```python
from build123d import *

# Parameters (mm, degrees)
F0_R     = 11
F1_DEPTH = 3.5
F2_R     = 5
F3_DEPTH = 1.5
F4_R     = 5
F5_DEPTH = 10
F6_R     = 4
F7_DEPTH = 25.4
F8_R     = 1.75
F9_DEPTH = 25.4
F10_SIZE = 0.381
F11_SIZE = 0.381


with BuildPart() as f1:
    # F0 (on Front) → F1 (new body)
    with BuildSketch(Plane.XZ):
        Circle(F0_R)
    extrude(amount=F1_DEPTH)

    # F2 (on face) → F3 (join)
    with BuildSketch(Plane.XZ.offset(3.5)):
        Circle(F2_R)
    extrude(amount=F3_DEPTH)

    # F4 (on face) → F5 (join)
    with BuildSketch(Plane(origin=(0, 0, 0), x_dir=(-1, 0, 0), z_dir=(0, 1, 0))):
        Circle(F4_R)
    extrude(amount=F5_DEPTH)

    # F6 (on face) → F7 (cut)
    with BuildSketch(Plane.XZ.offset(5)):
        Circle(F6_R)
    extrude(amount=-F7_DEPTH, mode=Mode.SUBTRACT)

    # F8 (on face) → F9 (cut)
    with BuildSketch(Plane.XZ.offset(3.5)):
        with Locations((-8, 0)):
            Circle(F8_R)
        with Locations((8, 0)):
            Circle(F8_R)
        with Locations((0, 8)):
            Circle(F8_R)
        with Locations((0, -8)):
            Circle(F8_R)
    extrude(amount=-F9_DEPTH, mode=Mode.SUBTRACT)

    # F10
    f10_edges = [f1.edges().sort_by_distance(p)[0] for p in [
        (11, -1.75, 0),
        (-11, 0, 0),
        (-11, -3.5, 0),
    ]]
    chamfer(f10_edges, length=F10_SIZE)

    # F11
    f11_edges = [f1.edges().sort_by_distance(p)[0] for p in [
        (5, 10, 0),
        (-5, -5, 0),
    ]]
    chamfer(f11_edges, length=F11_SIZE)


solid = f1.part
```
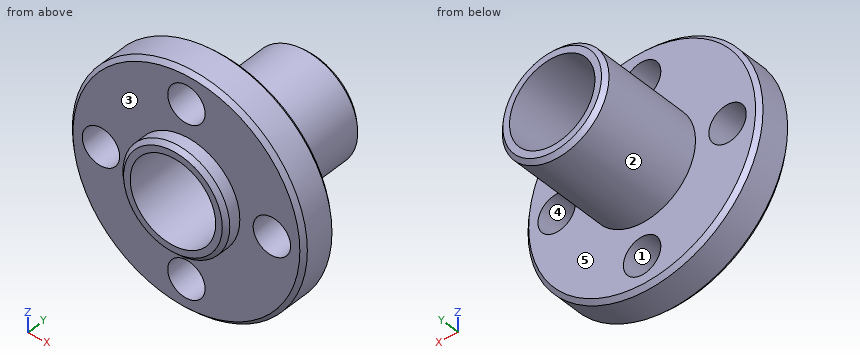
Source: CAD feature listing. Evaluate the final solid. Frame: model axes, mm. Face numbers are marked on the shaded views. A direction names the side the tool comes from. Round coordinates to 2 decimals unless told otherwise and drop trailing zeros. Write each loop counter-clockwise with the first axis right and the second up, starting at its lowest first coordinate (ties: lowest second). Pieces come first, ordered by that corner, then holes. Notation, with made-up numbers: M 7,57.25 L 28,57.25 A13 ccw 28,69.25 Z; hole C -26.75,10.25 d7. An arc over 180 degrees is marked long. Use CSV: the item, a comma, the result in double quotes. Start each with the question number.
Q1. Access query for the marked faces 4 and 5. Directions: +Z, -Z, +X, -X, +Y, -Y. A direction counts if a zero-diameter tool reaches every point of the face in a straight line with its end or side. Return the directions, or none.
Q2. Cut plane D-D on y = 5.75. Output: boundary loops of the cut face in (x, z), plus the area to 3 significant figures.
Q3. Line query: line 1 (Z direction, x = 0, y = -1.85); line 2 (Y direction, x = -5.75, z = 2); line 3 (Z direction, x = -8, y = -2.35). Output: solid intervals per line, ascending. Write a range as from..to.
Q4. Pull-direction query (Z, two-part tool) for the marked faces 1, 2 and 3; classes: +Z half, -Z half, draft (parallel to the pull), parting line (faces both ways), or undercut.
Q5. Cut plane A-A on z = 0. Count the separate pieces of the cut face and the enclosed holes in it, plus the area to 3 significant figures.
Q6. Cut plane C-C on y = -2.75. Output: boundary loops of the cut face in (x, z), plus the area to 3 significant figures.
Q7. First-contact query: P1, Ø5.5, axis at x = 0, z = -8, coming from the -Y side; P2, Ø1.5, axis at y = 5, z = 3, coming from the -X side; P3, Ø1.5, axis at x = -3, y = 5.5, coming from the +Z side. Flat tips, straight axial feed; report the tip coordinate or a pass-through.
Results found:
1,face 4,"+Y, -Y"
1,face 5,"+Y"
2,outline,"C 0,0 d10; hole C 0,0 d8"
2,area,"28.3 mm^2"
3,line 1,"-11..-9.75, -6.25..-4, 4..6.25, 9.75..11"
3,line 2,"-3.5..0"
3,line 3,"-7.55..-1.75, 1.75..7.55"
4,face 1,"undercut"
4,face 2,"parting line"
4,face 3,"draft"
5,separate pieces,"4"
5,enclosed holes,"0"
5,area,"46.9 mm^2"
6,outline,"C 0,0 d22; hole C -8,0 d3.5; hole C 0,0 d8; hole C 0,-8 d3.5; hole C 0,8 d3.5; hole C 8,0 d3.5"
6,area,"291 mm^2"
7,P1,"y = -3.5"
7,P2,"x = -4.47"
7,P3,"z = 4.47"
